Design review of the part built by this model. Coordinates are the model's own, in mm. Face numbers are marked on the shaded views. A direction names the side the tool comes from. Give positions to 0.01 mm unless a question says otherwise; leave off trailing zeros. Write each loop counter-clockwise with the first axis right and the second up, starting at its lowest first coordinate (ties: lowest second). Pieces come first, ordered by that corner, then holes. Notation, with made-up numbers: M 65,55 L 111,55 A24 ccw 111,89 Z; hole C -11,-18.75 d5. An arc over 180 degrees is marked long. Answer in a Markdown table with one row per item.
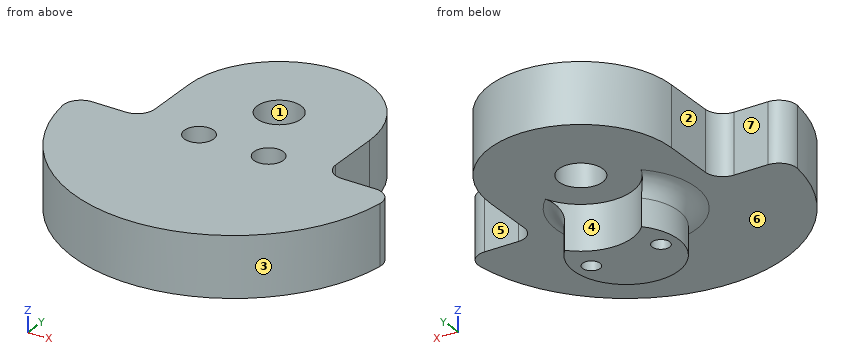
Autodesk Inventor part; units mm, degrees
ref_plane "YZ Plane" through (0, 0, 0) normal (1, 0, 0) x (0, 1, 0)
ref_plane "XZ Plane" through (0, 0, 0) normal (0, 1, 0) x (-1, 0, 0)
ref_plane "XY Plane" through (0, 0, 0) normal (0, 0, 1) x (1, 0, 0)
sketch "Sketch1" plane through (0, 0, 0) normal (0, 0, 1) x (1, 0, 0)
  circle A0 centre (0, 12.7) radius 3.9878
  circle A1 centre (-6.35, 0) radius 1.5875
  circle A2 centre (6.35, 0) radius 1.5875
  circle A3 centre (0, 0) radius 9.525
  arc A4 (-28.992, -3.5622) -> (28.992, -3.5622) centre (0, 0) ccw
  line L0 (-16.51, 12.7) -> (-16.51, 3.175)
  line L1 (16.51, 12.7) -> (16.51, 3.175)
  line L2 (19.685, 0) -> (25.8407, 0)
  line L3 (-19.685, 0) -> (-25.8407, 0)
  arc A5 (16.51, 12.7) -> (-16.51, 12.7) centre (0, 12.7) ccw
  arc A6 (-25.8407, 0) -> (-28.992, -3.5622) centre (-25.8407, -3.175) ccw
  arc A7 (-19.685, 0) -> (-16.51, 3.175) centre (-19.685, 3.175) ccw
  arc A8 (16.51, 3.175) -> (19.685, 0) centre (19.685, 3.175) ccw
  arc A9 (28.992, -3.5622) -> (25.8407, 0) centre (25.8407, -3.175) ccw
  circle A10 centre (6.35, 0) radius 2.667
  circle A11 centre (-6.35, 0) radius 2.667
  circle A12 centre (0, 12.7) radius 9.398
  point P0 (-9.525, 0)
  point P1 (9.525, 0)
  point P2 (-16.51, -24.0966)
  point P3 (16.51, -24.0966)
  point P4 (-29.21, 0)
  point P5 (29.21, 0)
  point P6 (-2.077, 9.2958)
  point P7 (2.077, 9.2958)
  point P8 (7.0137, 6.4446)
  point P9 (-7.0137, 6.4446)
  dimension "d20" = 7.9756
  dimension "d44" = 3.175
  dimension "d51" = 5.334
  dimension "d52" = 5.334
  dimension "d57" = 18.796
extrude "Extrusion9" add sketch "Sketch1" along normal blind 19.05 contours A0 A3 | A0 A3 A12 | A3 A0 | A0 A3 A12 | A12 A3 | A1 | A2 | A6 L3 A7 L0 A5 L1 A8 L2 A9 A4 | A10 | A11
extrude "Extrusion10" cut sketch "Sketch1" along normal blind 8.128 contours A0 A3 | A0 A3 A12 | A3 A0 | A0 A3 A12 | A6 L3 A7 L0 A5 L1 A8 L2 A9 A4
extrude "Extrusion11" cut sketch "Sketch1" along normal blind 38.1 contours A0 A3 | A3 A0
extrude "Extrusion12" cut sketch "Sketch1" along normal blind 38.1 contours A1 | A2 | A10 | A11
extrude "Extrusion13" add sketch "Sketch1" along normal blind 9.525 contours A10 | A11
fillet "Fillet2" radius 3.175 1 edges at (0, -9.525, 8.128)
properties part number "Crank on Crankshaft_3DPrint"
1) Add section B-B (z = 13.5). Write out the cut boundary in (x, y) (3 decimals).
Geometry says:
| item | result |
|---|---|
| outline | M -28.992,-3.562 A29.21 ccw 28.992,-3.562 A3.175 ccw 25.841,0 L 19.685,0 A3.175 cw 16.51,3.175 L 16.51,12.7 A16.51 ccw -16.51,12.7 L -16.51,3.175 A3.175 cw -19.685,0 L -25.841,0 A3.175 ccw Z; hole C -6.35,0 d5.334; hole C 0,12.7 d7.976; hole C 6.35,0 d5.334 |
2) Add section D-D (y = -24). Write out the cut boundary in (x, z), and give its area (3 significant figures).
Geometry says:
| item | result |
|---|---|
| outline | M -16.65,8.13 L 16.65,8.13 L 16.65,19.05 L -16.65,19.05 Z |
| area | 364 mm^2 |
3) Add section A-A (x = 0). Write out the cut boundary in (y, z) (3 decimals), and give its area (3 significant figures).
Geometry says:
| item | result |
|---|---|
| outline | M -29.21,8.128 L -12.7,8.128 A3.175 cw -9.525,4.953 L -9.525,0 L 3.302,0 L 3.302,8.128 L 8.712,8.128 L 8.712,19.05 L -29.21,19.05 Z; M 16.688,8.128 L 29.21,8.128 L 29.21,19.05 L 16.688,19.05 Z |
| area | 657 mm^2 |
4) To check wall thickness, follow probe 1 along Y at (x, z) = (0, 14.25); probe 2 along Z at (x, y) = (-8.5, -16.5); probe 3 along Y at (x, z) = (6, 4). State the ranges of each line that lie inside material, in increasing order. Write a range as [from, to].
Geometry says:
| item | result |
|---|---|
| probe 1 | [-29.21, 8.71], [16.69, 29.21] |
| probe 2 | [8.13, 19.05] |
| probe 3 | [-7.4, -1.55], [1.55, 5.47] |
5) The part is to be moulded in two halves that separate along X. For the marked faces 1, 2 and 3, say which applies: released by +X, released by -X, zero draft, split by the parting line, or undercut.
Geometry says:
| item | result |
|---|---|
| face 1 | undercut |
| face 2 | released by -X |
| face 3 | split by the parting line |
6) Add section C-C (z = 6). Count the separate pieces of the cut face and the enclosed holes in it, and give its area (3 significant figures).
Geometry says:
| item | result |
|---|---|
| separate pieces | 1 |
| enclosed holes | 2 |
| area | 217 mm^2 |
7) Insertion check: P1, Ø2, axis at y = -3.5, z = 12, coming from the -X side; P2, Ø3, axis at x = -22, z = 14.5, coming from the +Y side; P3, Ø3, axis at y = 6.5, z = 13, coming from the -X side; P4, Ø1.6, axis at x = 7.5, y = 0, coming from the +Z side (3 decimals). Each pin has a flat end and moves straight along its axis. Give the tip position at first contact, or say it passes through.
Geometry says:
| item | result |
|---|---|
| P1 | x = -29.02 |
| P2 | y = 0 |
| P3 | x = -16.51 |
| P4 | z = 9.525 |
8) For the marked faces 4, 5, 6 and 7, list the 3-axis set-ups (+Z, -Z, +X, -X, +Y, -Y) from which the entire face can be reached by the end or side of a thin tool; tool diameter is ignored.
Geometry says:
| item | result |
|---|---|
| face 4 | -Z, +Y |
| face 5 | +Z, -Z, +X, +Y |
| face 6 | -Z |
| face 7 | +Z, -Z, -X, +Y |
